Read the model definition and answer for the solid it produces. Units are mm, in the model's axes. A direction names the side the tool comes from. Coordinates: 2 decimals unless noted, no trailing zeros. Loops run counter-clockwise (first coordinate to the right, second up) from the corner with the lowest first, then second, coordinate; pieces in that order, holes last. Notation, with made-up numbers: (-16, 78) - (6, 78) arc R15 cw to (6, 83) - close; hole circle Ø3 at (37.5, -14). An arc over 180 degrees is marked (long way). One line per item, written item: value. Start each with the question number.
Autodesk Inventor part; units mm, degrees
ref_plane "YZ Plane" through (0, 0, 0) normal (1, 0, 0) x (0, 1, 0)
ref_plane "XZ Plane" through (0, 0, 0) normal (0, 1, 0) x (-1, 0, 0)
ref_plane "XY Plane" through (0, 0, 0) normal (0, 0, 1) x (1, 0, 0)
sketch "Sketch1" plane through (0, 0, 0) normal (0, 0, 1) x (1, 0, 0)
  line L0 (-27.5, -45) -> (27.5, -45)
  line L1 (27.5, -45) -> (27.5, 45)
  line L2 (27.5, 45) -> (-27.5, 45)
  line L3 (-27.5, 45) -> (-27.5, -45)
  line L4 (-27.5, -45) -> (27.5, 45) construction
  line L5 (27.5, -45) -> (-27.5, 45) construction
  line L6 (-24.5, -42) -> (24.5, -42)
  line L7 (24.5, -42) -> (24.5, 42)
  line L8 (24.5, 42) -> (-24.5, 42)
  line L9 (-24.5, 42) -> (-24.5, -42)
  line L10 (-24.5, -42) -> (24.5, 42) construction
  line L11 (24.5, -42) -> (-24.5, 42) construction
  point P0 (0, 0)
  dimension "d0" = 55
  dimension "d1" = 90
  dimension "d2" = 49
  dimension "d3" = 84
extrude "Extrusion1" add sketch "Sketch1" along normal blind 50
sketch "Sketch2" plane through (-27.5, -45, 0) normal (0, -1, 0) x (1, 0, 0)
  circle A0 centre (15, 40) radius 2.75
  circle A1 centre (40, 40) radius 2.75
  circle A2 centre (15, 10) radius 2.75
  circle A3 centre (40, 10) radius 2.75
  line L0 (55, 0) -> (55, 50)
  line L1 (0, 50) -> (55, 50)
  line L2 (0, 0) -> (55, 0)
  line L3 (0, 0) -> (0, 50)
  point P0 (27.5, 0)
  dimension "d6" = 5.5
  dimension "d7" = 5.5
  dimension "d8" = 5.5
  dimension "d9" = 5.5
  dimension "d10" = 15
  dimension "d11" = 10
  dimension "d12" = 15
  dimension "d13" = 10
  dimension "d14" = 10
  dimension "d15" = 15
  dimension "d16" = 15
  dimension "d17" = 10
extrude "Extrusion2" cut sketch "Sketch2" against normal blind 97.625 contours A0 | A1 | A2 | A3
sketch "Sketch3" plane through (27.5, -45, 0) normal (1, 0, 0) x (0, 0, -1)
  circle A0 centre (-39.023, 57.7) radius 2.25
  circle A1 centre (-13.623, 57.7) radius 2.25
  circle A2 centre (-39.023, 32.3) radius 2.25
  circle A3 centre (-13.623, 32.3) radius 2.25
  line L0 (0, 90) -> (-50, 90)
  line L1 (0, 0) -> (0, 90)
  point P0 (0, 45)
  dimension "d20" = 4.5
  dimension "d21" = 4.5
  dimension "d22" = 4.5
  dimension "d23" = 4.5
  dimension "d24" = 25.4
  dimension "d25" = 25.4
  dimension "d26" = 25.4
  dimension "d27" = 25.4
  dimension "d29" = 25.4
  dimension "d30" = 25.4
  dimension "d31" = 32.3
  dimension "d32" = 13.623
extrude "Extrusion3" cut sketch "Sketch3" against normal blind 60
properties part number "Front Motor Connector"
1) Section C-C, the plane x = 12.5 is taken. Determine the outline of the cut face in (y, z).
2) Section D-D, the plane y = -3.5 is taken. Determine the outline of the cut face in (x, z).
3) For faces 4 (the cylindrical face through (-11.02, -43.52, 12.32)), 5 (the flat face through (0, 42, 25)), determine the directions among +Z, -Z, +X, -X, +Y, -Y from which every point of the face is accessible in a straight line to the end or side of a thin tool.
4) Determine the mould class of faces 1 (the flat face through (-27.5, 1, 25)), 2 (the cylindrical face through (-11.02, 43.48, 12.32)), 3 (the cylindrical face through (-25.98, 11.33, 40.81)) for opening direction X: released by +X, released by -X, zero draft, split by the parting line, or undercut.
5) Section A-A, the plane y = 12.7 is taken. Determine the outline of the cut face in (x, z).
6) Straight lines are drawn through the part: L1, parallel to Y at x = -19, z = 12.5; L2, parallel to X at y = -13, z = 29; L3, parallel to Z at x = 12.5, y = -43.6. For each, find the intervals that lie inside material, in ascending order.
7) Section B-B, the plane z = 10 is taken. Determine the outline of the cut face in (x, y).
Answer below:
1. outline: (-45, 0) - (-42, 0) - (-42, 7.25) - (-45, 7.25) - close; (-45, 12.75) - (-42, 12.75) - (-42, 37.25) - (-45, 37.25) - close; (-45, 42.75) - (-42, 42.75) - (-42, 50) - (-45, 50) - close; (42, 0) - (45, 0) - (45, 7.25) - (42, 7.25) - close; (42, 12.75) - (45, 12.75) - (45, 37.25) - (42, 37.25) - close; (42, 42.75) - (45, 42.75) - (45, 50) - (42, 50) - close
2. outline: (-27.5, 0) - (-24.5, 0) - (-24.5, 50) - (-27.5, 50) - close; (24.5, 0) - (27.5, 0) - (27.5, 50) - (24.5, 50) - close
3. face 4: +Y, -Y
3. face 5: +Z, -Z
4. face 1: released by -X
4. face 2: undercut
4. face 3: zero draft
5. outline: (-27.5, 0) - (-24.5, 0) - (-24.5, 11.37) - (-27.5, 11.37) - close; (-27.5, 15.87) - (-24.5, 15.87) - (-24.5, 36.77) - (-27.5, 36.77) - close; (-27.5, 41.27) - (-24.5, 41.27) - (-24.5, 50) - (-27.5, 50) - close; (24.5, 0) - (27.5, 0) - (27.5, 11.37) - (24.5, 11.37) - close; (24.5, 15.87) - (27.5, 15.87) - (27.5, 36.77) - (24.5, 36.77) - close; (24.5, 41.27) - (27.5, 41.27) - (27.5, 50) - (24.5, 50) - close
6. L1: -45 to -42, 42 to 45
6. L2: -27.5 to -24.5, 24.5 to 27.5
6. L3: 0 to 7.25, 12.75 to 37.25, 42.75 to 50
7. outline: (-27.5, -45) - (-15.25, -45) - (-15.25, -42) - (-24.5, -42) - (-24.5, 42) - (-15.25, 42) - (-15.25, 45) - (-27.5, 45) - close; (-9.75, -45) - (9.75, -45) - (9.75, -42) - (-9.75, -42) - close; (-9.75, 42) - (9.75, 42) - (9.75, 45) - (-9.75, 45) - close; (15.25, -45) - (27.5, -45) - (27.5, 45) - (15.25, 45) - (15.25, 42) - (24.5, 42) - (24.5, -42) - (15.25, -42) - close
